```python
from build123d import *

# Parameters (mm, degrees)
F0_W     = 40
F0_H     = 20
F0_W_2   = 35.4
F0_H_2   = 15.4
F1_DEPTH = 900


with BuildPart() as f1:
    # F0 (on Right) → F1 (new body)
    with BuildSketch(Plane.YZ):
        Rectangle(F0_W, F0_H)
        Rectangle(F0_W_2, F0_H_2, mode=Mode.SUBTRACT)
    extrude(amount=-F1_DEPTH)


solid = f1.part
```
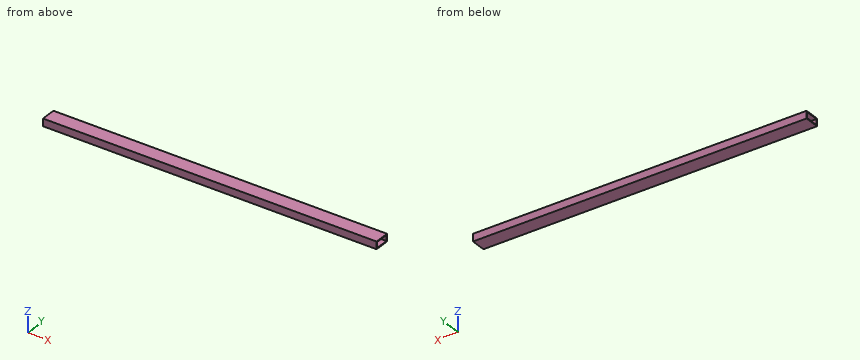
Source: CAD feature listing. Evaluate the final solid. Frame: model axes, mm. Round coordinates to 2 decimals unless told otherwise and drop trailing zeros. Order: outer loops, then holes, each group sorted by start corner. A loop starts at its lowest first (then second) coordinate and runs counter-clockwise, first axis right, second up. Notation, with made-up numbers: (50, 66.25) -> (88, 66.25) arc R11 ccw to (88, 77.25) -> close; hole circle Ø3 at (63, -9). An arc over 180 degrees is marked (long way). One line per item, written item: value. Start each with the question number.
Q1. Pin query (flat end, axial travel): pin 1 (12 mm diameter, centred on y = 10.5, z = 1, fed in from +X). Return the tip coordinate at first contact, or that it passes through.
Q2. Section query C-C (x = -534.5). Return the cut outline in (y, z).
Q3. Material intervals for probe 1 along Z at (x, y) = (-191, -13.5); probe 2 along Y at (x, z) = (-821, -6.25), sorted ascending.
Q4. Section query B-B (z = 0.75). Return the cut outline in (x, y), plus the area to 3 significant figures.
Q5. Section query A-A (y = 11). Return the cut outline in (x, z).
Findings below:
1. pin 1: through
2. outline: (-20, -10) -> (20, -10) -> (20, 10) -> (-20, 10) -> close; hole (-17.7, -7.7) -> (17.7, -7.7) -> (17.7, 7.7) -> (-17.7, 7.7) -> close
3. probe 1: -10 to -7.7, 7.7 to 10
3. probe 2: -20 to -17.7, 17.7 to 20
4. outline: (-900, -20) -> (0, -20) -> (0, -17.7) -> (-900, -17.7) -> close; (-900, 17.7) -> (0, 17.7) -> (0, 20) -> (-900, 20) -> close
4. area: 4,140 mm²
5. outline: (-900, -10) -> (0, -10) -> (0, -7.7) -> (-900, -7.7) -> close; (-900, 7.7) -> (0, 7.7) -> (0, 10) -> (-900, 10) -> close
